CAD build for the part. Positions are in the model's coordinates, mm. Give positions to 0.01 mm unless a question says otherwise; leave off trailing zeros. Loops run counter-clockwise (first coordinate to the right, second up) from the corner with the lowest first, then second, coordinate; pieces in that order, holes last. Notation, with made-up numbers: (24.5, 45) - (53.5, 45) arc R21 cw to (53.5, 61) - close; hole circle Ø9 at (28.25, 72.5). An arc over 180 degrees is marked (long way). Return JSON: item names as keys, results as strings.
from build123d import *

# Parameters (mm, degrees)
SKETCH_R  = 1.5
PAD_DEPTH = 10


with BuildPart() as part:
    # Sketch → Pad (new body)
    with BuildSketch(Plane.XY):
        with BuildLine():
            ThreePointArc((-4.788282, 13.155697), (-6.581299, 9.310558), (-2.736161, 7.517541))
            ThreePointArc((2.736161, 7.517541), (0, 8), (-2.736161, 7.517541))
            ThreePointArc((2.736161, 7.517541), (6.581299, 9.310558), (4.788282, 13.155697))
            ThreePointArc((4.788282, 13.155697), (0, 14), (-4.788282, 13.155697))
        make_face()
        with Locations((-3.762222, 10.336619)):
            Circle(SKETCH_R, mode=Mode.SUBTRACT)
        with Locations((3.762222, 10.336619)):
            Circle(SKETCH_R, mode=Mode.SUBTRACT)
        with Locations((0, 11)):
            Circle(SKETCH_R, mode=Mode.SUBTRACT)
    extrude(amount=PAD_DEPTH)


solid = part.part
1. Cut at D-D, the plane z = 8.5. Write the cut outline in (x, y).
Values follow:
{"outline": "(-4.79, 13.16) arc R3 ccw to (-2.74, 7.52) arc R8 cw to (2.74, 7.52) arc R3 ccw to (4.79, 13.16) arc R14 ccw to start; hole circle Ø3 at (-3.76, 10.34); hole circle Ø3 at (0, 11); hole circle Ø3 at (3.76, 10.34)"}
2. Drill centre lines: probe 1 along X at (y, z) = (11.25, 9.5); probe 2 along X at (y, z) = (9, 8.25); probe 3 along X at (y, z) = (9.75, 4.5). Where is each one in solid material? Low to high.
Values follow:
{"probe 1": "x = -6.62 to -4.95, -2.57 to -1.48, 1.48 to 2.57, 4.95 to 6.62", "probe 2": "x = -6.45 to -4.44, -3.08 to 3.08, 4.44 to 6.45", "probe 3": "x = -6.7 to -5.14, -2.38 to -0.83, 0.83 to 2.38, 5.14 to 6.7"}
3. Cut at A-A, the plane x = 0. Write the cut outline in (y, z).
Values follow:
{"outline": "(8, 0) - (9.5, 0) - (9.5, 10) - (8, 10) - close; (12.5, 0) - (14, 0) - (14, 10) - (12.5, 10) - close"}
4. Cut at B-B, the plane y = 9. Write the cut outline in (x, z).
Values follow:
{"outline": "(-6.45, 0) - (-4.44, 0) - (-4.44, 10) - (-6.45, 10) - close; (-3.08, 0) - (3.08, 0) - (3.08, 10) - (-3.08, 10) - close; (4.44, 0) - (6.45, 0) - (6.45, 10) - (4.44, 10) - close"}
5. Cut at C-C, the plane y = 11. Write the cut outline in (x, z).
Values follow:
{"outline": "(-6.69, 0) - (-5.11, 0) - (-5.11, 10) - (-6.69, 10) - close; (-2.42, 0) - (-1.5, 0) - (-1.5, 10) - (-2.42, 10) - close; (1.5, 0) - (2.42, 0) - (2.42, 10) - (1.5, 10) - close; (5.11, 0) - (6.69, 0) - (6.69, 10) - (5.11, 10) - close"}
6. Drop flat-ended pins along their axis: P1, Ø1.5, axis at x = 3, z = 1, coming from the +Y side; P2, Ø3.5, axis at x = 0, y = 11, coming from the -Z side. Give the stop position or say it passes through.
Values follow:
{"P1": "stops at y = 13.82", "P2": "stops at z = 0"}
7. Pull direction X, two halves, no side cores. Call faces 1 (the face through (0, 9, 10)), 2 (the face through (0, 8, 5)), 3 (the face through (4.57, 11.6, 4.93)), 4 (the face through (0, 14, 5)): +X half, -X half, draft (parallel to the pull), parting line (faces both ways), or undercut.
Values follow:
{"face 1": "draft", "face 2": "undercut", "face 3": "undercut", "face 4": "parting line"}
